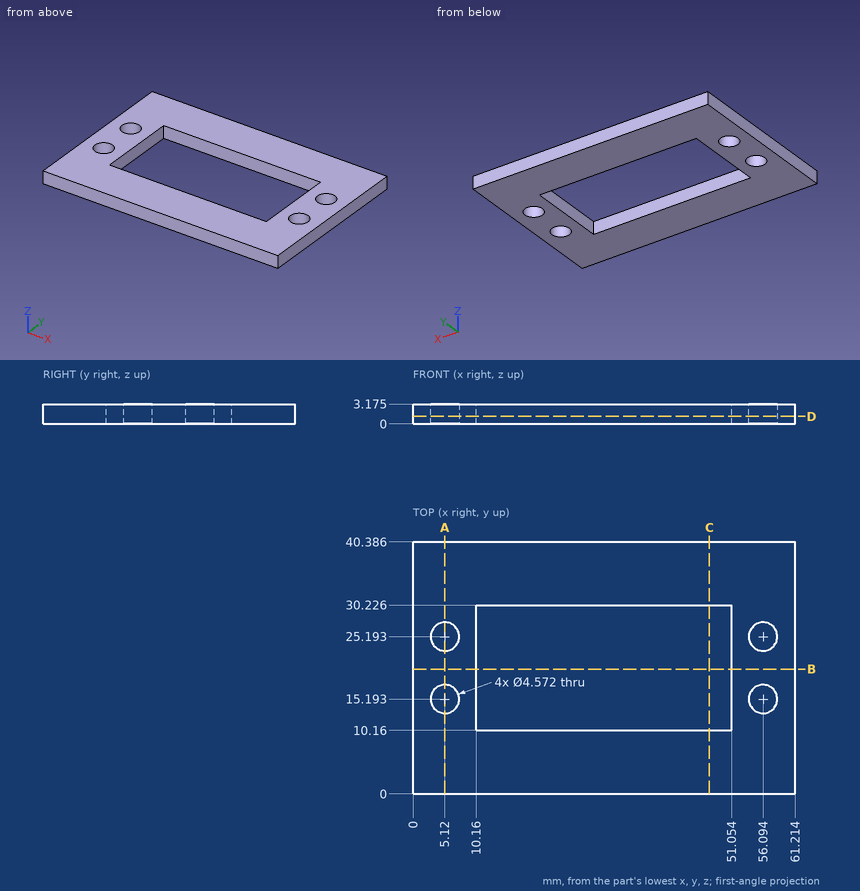
Print and shaded views of the part. All mm, measured from the part's lowest x, y and z. Round coordinates to 2 decimals unless told otherwise and drop trailing zeros. Order: outer loops, then holes, each group sorted by start corner. A loop starts at its lowest first (then second) coordinate and runs counter-clockwise, first axis right, second up.
Q1. Slice it at D-D (z = 1.2). Write the cut outline in (x, y), and give its area (3 significant figures).
Q2. Slice it at A-A (x = 5.12). Write the cut outline in (y, z) (3 decimals).
Q3. Slice it at B-B (y = 20). Write the cut outline in (x, z) (3 decimals).
Q4. Slice it at C-C (x = 47.5). Write the cut outline in (y, z) (3 decimals).
Q5. Drop flat-ended pins along their axis: pin 1 (1.6 mm diameter, centred on y = 17.5, z = 2, fed in from -X); pin 2 (4 mm diameter, centred on x = 5.12, y = 15.193, fed in from +Z). Give the stop position or say it passes through.
Q6. Wall check: L1, parallel to Y at x = 5.12, z = 2.45; L2, parallel to X at y = 25, z = 2.65; L3, parallel to Y at x = 29.5, z = 2.6. Give the ranges that are in metal, low to high.
Results below:
1. outline: (0, 0) - (61.21, 0) - (61.21, 40.39) - (0, 40.39) - close; hole circle Ø4.57 at (5.12, 15.19); hole circle Ø4.57 at (5.12, 25.19); hole (10.16, 10.16) - (51.05, 10.16) - (51.05, 30.23) - (10.16, 30.23) - close; hole circle Ø4.57 at (56.09, 15.19); hole circle Ø4.57 at (56.09, 25.19)
1. area: 1,590 mm2
2. outline: (0, 0) - (12.907, 0) - (12.907, 3.175) - (0, 3.175) - close; (17.479, 0) - (22.907, 0) - (22.907, 3.175) - (17.479, 3.175) - close; (27.479, 0) - (40.386, 0) - (40.386, 3.175) - (27.479, 3.175) - close
3. outline: (0, 0) - (10.16, 0) - (10.16, 3.175) - (0, 3.175) - close; (51.054, 0) - (61.214, 0) - (61.214, 3.175) - (51.054, 3.175) - close
4. outline: (0, 0) - (10.16, 0) - (10.16, 3.175) - (0, 3.175) - close; (30.226, 0) - (40.386, 0) - (40.386, 3.175) - (30.226, 3.175) - close
5. pin 1: stops at x = 0
5. pin 2: passes through
6. L1: y = 0 to 12.91, 17.48 to 22.91, 27.48 to 40.39
6. L2: x = 0 to 2.84, 7.4 to 10.16, 51.05 to 53.82, 58.37 to 61.21
6. L3: y = 0 to 10.16, 30.23 to 40.39
